```python
from build123d import *

# Parameters (mm, degrees)
F1_DEPTH             = 50
F1_DEPTH_BACK        = 6
F2_DEPTH             = 44
F5_D                 = 4.4958
F5_CSINK_D           = 9.1186
F5_CSINK_ANGLE       = 82
F5_ON_F3_D           = 4.4958
F5_ON_F3_CSINK_D     = 9.1186
F5_ON_F3_CSINK_ANGLE = 82
F6_R                 = 15
F7_R                 = 5


with BuildPart() as f1:
    # F0 (on Top) → F1 (new body, two sides)
    with BuildSketch(Plane.XY) as f1_sk:
        Polygon((-8, -60), (0, -60), (0, 0), (60, 0), (60, 8), (-8, 8), align=None)
        Polygon((19.75, -19.75), (19.75, -60), (25.75, -60), (25.75, -25.75), (60, -25.75), (60, -19.75), align=None)
        Polygon((0, 0), (0, -60), (19.75, -60), (19.75, -19.75), (60, -19.75), (60, 0), align=None)
    extrude(amount=F1_DEPTH)
    extrude(f1_sk.sketch, amount=-F1_DEPTH_BACK)

    # F0 (on Top) → F2 (cut)
    with BuildSketch(Plane.XY):
        Polygon((0, 0), (0, -60), (19.75, -60), (19.75, -19.75), (60, -19.75), (60, 0), align=None)
    extrude(amount=F2_DEPTH, mode=Mode.SUBTRACT)

    # F5 (through all)
    with Locations(Plane(origin=(-8, 0, 0), x_dir=(0, -1, 0), z_dir=(-1, 0, 0))):
        with Locations((8.875, 36), (8.875, 8)):
            CounterSinkHole(F5_D / 2, F5_CSINK_D / 2, counter_sink_angle=F5_CSINK_ANGLE)

    # F5 on F3 (through all)
    with Locations(Plane(origin=(0, 8, 0), x_dir=(-1, 0, 0), z_dir=(0, 1, 0))):
        with Locations((-9.875, 29), (-9.875, 15)):
            CounterSinkHole(F5_ON_F3_D / 2, F5_ON_F3_CSINK_D / 2, counter_sink_angle=F5_ON_F3_CSINK_ANGLE)

    # F6
    f6_edges = [f1.edges().sort_by_distance(p)[0] for p in [
        (25.75, -25.75, 22),
    ]]
    fillet(f6_edges, radius=F6_R)

    # F7
    f7_edges = [f1.edges().sort_by_distance(p)[0] for p in [
        (25.75, -50.375, 50),
        (30.143398, -30.143398, 50),
        (8.875, -60, 50),
        (50.375, -25.75, 50),
        (-8, -26, 50),
        (60, -8.875, 50),
        (26, 8, 50),
        (25.75, -50.375, -6),
        (30.143398, -30.143398, -6),
        (8.875, -60, -6),
        (50.375, -25.75, -6),
        (-8, -26, -6),
        (60, -8.875, -6),
        (26, 8, -6),
        (60, -25.75, 22),
        (60, 8, 22),
        (25.75, -60, 22),
        (-8, -60, 22),
        (-8, 8, 22),
    ]]
    fillet(f7_edges, radius=F7_R)


solid = f1.part
```
The listing builds one solid part. Answer for the finished solid, in the listing's coordinates (mm). A direction names the side the tool comes from. Coordinates: 2 decimals unless noted, no trailing zeros. Order: outer loops, then holes, each group sorted by start corner. A loop starts at its lowest first (then second) coordinate and runs counter-clockwise, first axis right, second up. Notation, with made-up numbers: M 53.5,70.5 L 101.5,70.5 A31 ccw 101.5,106.5 Z; hole C 63,-35.5 d7. An arc over 180 degrees is marked long. Answer as a JSON object with one key per item and string values. Group by question number.
1. Flat-ended cylindrical pins translate along their axes: P1, Ø5, axis at x = 9.875, z = 29, coming from the +Y side; P2, Ø7, axis at y = -8.875, z = 8, coming from the -X side; P3, Ø6, axis at y = -8.875, z = 36, coming from the -X side. Find the tip coordinate at first contact, or state that the pin passes through.
2. Section C-C on x = 10.5 is taken. State how many separate pieces and enclosed holes the cut face has, then the cut area to 3 significant figures.
3. Determine the mould class of faces 1 (the conical face through (9.363, 5.47, 12.696)), 2 (the flat face through (19, -19, -6)), 3 (the cylindrical face through (24.25, -47.78, -4.57)) for opening direction X: released by +X, released by -X, zero draft, split by the parting line, or undercut.
4. Section B-B on z = 15 is taken. Write down the section's boundary in (x, y).
5. Straight lines are drawn through the part: line 1 (X direction, y = -49, z = 29); line 2 (Y direction, x = 48.5, z = 10.5). For each, find the intervals that lie inside material, in ascending order.
6. Section A-A on y = -50 is taken. Write down the section's boundary in (x, z), then the cut area to 4 significant figures.
7. A tool of negligible diameter and unlimited length cuts with its end or side. For faces 4 (the flat face through (30, 0, 22)), 5 (the cylindrical face through (47.97, -24.25, -4.57)), 6 (the cylindrical face through (24.25, -47.78, 48.57)), 7 (the flat face through (23, -16, 44)), 8 (the cylindrical face through (-2.63, -7.67, 37.9)), from which of +Z, -Z, +X, -X, +Y, -Y can it reach the whole face along a straight path? Write none if from no direction.
Values follow:
{
 "1": {"P1": "y = 5.63", "P2": "x = -6.78", "P3": "x = -6.21"},
 "2": {"separate pieces": "3", "enclosed holes": "0", "area": "1,060 mm2"},
 "3": {"face 1": "undercut", "face 2": "zero draft", "face 3": "released by +X"},
 "4": {"outline": "M -8,-55 A5 ccw -3,-60 L 0,-60 L 0,0 L 7.63,0 L 7.63,5.34 L 5.32,8 L -3,8 A5 ccw -8,3 Z; M 12.12,0 L 60,0 L 60,3 A5 ccw 55,8 L 14.43,8 L 12.12,5.34 Z; M 19.75,-60 L 20.75,-60 A5 ccw 25.75,-55 L 25.75,-40.75 A15 cw 40.75,-25.75 L 55,-25.75 A5 ccw 60,-20.75 L 60,-19.75 L 19.75,-19.75 Z"},
 "5": {"line 1": "-8 to 0, 19.75 to 25.75", "line 2": "-25.75 to -19.75, 0 to 8"},
 "6": {"outline": "M -8,-1 A5 ccw -3,-6 L 20.75,-6 A5 ccw 25.75,-1 L 25.75,45 A5 ccw 20.75,50 L -3,50 A5 ccw -8,45 Z; hole M 0,0 L 19.75,0 L 19.75,44 L 0,44 Z", "area": "1,000 mm2"},
 "7": {"face 4": "+X", "face 5": "-Z, +X, -Y", "face 6": "+Z, +X, -Y", "face 7": "none", "face 8": "+X, -X"}
}
